Source: CAD feature listing. Evaluate the final solid. Frame: model axes, mm. A direction names the side the tool comes from. Give positions to 0.01 mm unless a question says otherwise; leave off trailing zeros. Write each loop counter-clockwise with the first axis right and the second up, starting at its lowest first coordinate (ties: lowest second). Pieces come first, ordered by that corner, then holes. Notation, with made-up numbers: (67, 43.25) -> (75, 43.25) arc R24 ccw to (75, 57.25) -> close; hole circle Ø8 at (28.5, -2.75). An arc over 180 degrees is marked (long way). Answer as a JSON object with one key per item and string values. Group by question number.
Item 1: Section query D-D on y = -2.5. Return the cut outline in (x, z), plus the area to 3 significant figures.
Item 2: Section query A-A on y = 1.25. Return the cut outline in (x, z).
Item 3: Access query for faces 1 (the face through (4.737, 1.26, 6.176)), 2 (the face through (5, -4.5, 11)), 3 (the face through (2, -3, 11)), 4 (the face through (-4, -1, 11)). Directions: +Z, -Z, +X, -X, +Y, -Y. A direction counts if a zero-diameter tool reaches every point of the face in a straight line with its end or side. Return the directions, or none.
Item 4: Section query C-C on y = -1.25. Return the cut outline in (x, z), plus the area to 3 significant figures.
Item 5: Pull-direction query (Z, two-part tool) for faces 5 (the face through (-4, 0.5, 18)), 6 (the face through (0.1, 0.2, 23)), 7 (the face through (0.1, 0.2, 0)), 8 (the face through (-3.783, 1.26, 16.524)); classes: pulls with the +Z half, pulls with the -Z half, needs draft (parallel to the pull), parting line crosses it, or undercut.
Item 6: Ray query, probe 1 along Z at (x, y) = (-4, 1.75); probe 2 along X at (y, z) = (-2.25, 18.75); probe 3 along X at (y, z) = (-0.75, 7). Return the intervals inside material, ascending. Write a range as from..to.
Item 7: Section query B-B on z = 17.5. Return the cut outline in (x, y).
Item 8: First-contact query: pin 1 Ø2.5 at (x, z) = (0, 16) entering from -Y; pin 2 Ø1.2 at (x, z) = (4, 17.5) entering from +Y. Flat tips, straight axial feed; report the tip coordinate or a pass-through.
from build123d import *

# Parameters (mm, degrees)
DODANIE_WYCI_GNI_CIE1_DEPTH = 23
SZKIC2_R                    = 1
WYTNIJ_WYCI_GNI_CIE1_DEPTH  = 1.5


with BuildPart() as part:
    # Szkic1 → Dodanie-wyciągnięcie1 (new body)
    with BuildSketch(Plane.XY):
        Polygon((0, 0), (0, 2), (-8.5, 2), (-8.5, -4.5), (-2, -4.5), (-2, -2.2), (-4, -2.2), (-4, 0), align=None)
    dodanie_wyci_gni_cie1 = extrude(amount=DODANIE_WYCI_GNI_CIE1_DEPTH)

    # Lustro1: Dodanie-wyciągnięcie1 across plane
    add(dodanie_wyci_gni_cie1.mirror(Plane(origin=(0, 0, 23), x_dir=(0, 0, 1), z_dir=(-1, 0, 0))))

    # Szkic2 → Wytnij-wyciągnięcie1 (cut)
    with BuildSketch(Plane(origin=(0, 2, 0), x_dir=(1, 0, 0), z_dir=(0, 1, 0))):
        with Locations(Location((-4, -5.5, 0), (0, 0, 180))):
            Circle(SZKIC2_R)
        with Locations(Location((4, -5.5, 0), (0, 0, 180))):
            Circle(SZKIC2_R)
        with Locations(Location((4, -17.5, 0), (0, 0, 180))):
            Circle(SZKIC2_R)
        with Locations(Location((-4, -17.5, 0), (0, 0, 180))):
            Circle(SZKIC2_R)
    extrude(amount=-WYTNIJ_WYCI_GNI_CIE1_DEPTH, mode=Mode.SUBTRACT)


solid = part.part
Worked answers:
{
 "1": {"outline": "(-8.5, 0) -> (-2, 0) -> (-2, 23) -> (-8.5, 23) -> close; (2, 0) -> (8.5, 0) -> (8.5, 23) -> (2, 23) -> close", "area": "299 mm^2"},
 "2": {"outline": "(-8.5, 0) -> (8.5, 0) -> (8.5, 23) -> (-8.5, 23) -> close; hole circle Ø2 at (-4, 5.5); hole circle Ø2 at (-4, 17.5); hole circle Ø2 at (4, 5.5); hole circle Ø2 at (4, 17.5)"},
 "3": {"face 1": "+Y", "face 2": "+Z, -Z, +X, -X, -Y", "face 3": "+Z, -Z, -Y", "face 4": "+Z, -Z"},
 "4": {"outline": "(-8.5, 0) -> (-4, 0) -> (-4, 23) -> (-8.5, 23) -> close; (4, 0) -> (8.5, 0) -> (8.5, 23) -> (4, 23) -> close", "area": "207 mm^2"},
 "5": {"face 5": "undercut", "face 6": "pulls with the +Z half", "face 7": "pulls with the -Z half", "face 8": "undercut"},
 "6": {"probe 1": "0..4.5, 6.5..16.5, 18.5..23", "probe 2": "-8.5..-2, 2..8.5", "probe 3": "-8.5..-4, 4..8.5"},
 "7": {"outline": "(-8.5, -4.5) -> (-2, -4.5) -> (-2, -2.2) -> (-4, -2.2) -> (-4, 0) -> (4, 0) -> (4, -2.2) -> (2, -2.2) -> (2, -4.5) -> (8.5, -4.5) -> (8.5, 2) -> (5, 2) -> (5, 0.5) -> (3, 0.5) -> (3, 2) -> (-3, 2) -> (-3, 0.5) -> (-5, 0.5) -> (-5, 2) -> (-8.5, 2) -> close"},
 "8": {"pin 1": "y = 0", "pin 2": "y = 0.5"}
}
